from build123d import *

# Parameters (mm, degrees)
EXTRUDE_1_DEPTH        = 5
SKETCH_1_4_OUTSIDE_W   = 152.016
SKETCH_1_4_OUTSIDE_H   = 122.016
SKETCH_1_4_OUTSIDE_R   = 1.7
SKETCH_1_4_OUTSIDE_R_2 = 1.6
CUT_EXTRUDE_3_DEPTH    = 84.683501662
SKETCH_2_W             = 7.5
SKETCH_2_H             = 25
EXTRUDE_2_DEPTH        = 20
FILLET_1_R             = 2
SKETCH_6_R             = 1.6
CUT_EXTRUDE_4_DEPTH    = 7.5
SKETCH_7_R             = 1.6
CUT_EXTRUDE_5_DEPTH    = 134.554368416


with BuildPart() as part:
    # 스케치1 → 보스-돌출1 (new body)
    with BuildSketch(Plane.XY):
        with BuildLine():
            Line((-57.749377558, 34.859778143), (52.250622442, 34.859778143))
            ThreePointArc((52.250622442, 34.859778143), (55.786156348, 33.395312049), (57.250622442, 29.859778143))
            Line((57.250622442, 29.859778143), (57.250622442, -50.140221857))
            ThreePointArc((57.250622442, -50.140221857), (55.786156348, -53.675755763), (52.250622442, -55.140221857))
            Line((52.250622442, -55.140221857), (-57.749377558, -55.140221857))
            ThreePointArc((-57.749377558, -55.140221857), (-61.284911464, -53.675755763), (-62.749377558, -50.140221857))
            Line((-62.749377558, -50.140221857), (-62.749377558, 29.859778143))
            ThreePointArc((-62.749377558, 29.859778143), (-61.284911464, 33.395312049), (-57.749377558, 34.859778143))
        make_face()
    extrude(amount=-EXTRUDE_1_DEPTH)

    # 스케치1<4> outside → 컷-돌출3 (cut, through all)
    # profile 1 of 11: a face of its own
    with BuildSketch(Plane.XY):
        with Locations((-2.749, -10.14)):
            Rectangle(SKETCH_1_4_OUTSIDE_W, SKETCH_1_4_OUTSIDE_H)
        with BuildLine():
            Line((-57.749377558, 34.859778143), (52.250622442, 34.859778143))
            ThreePointArc((52.250622442, 34.859778143), (55.786156348, 33.395312049), (57.250622442, 29.859778143))
            Line((57.250622442, 29.859778143), (57.250622442, -50.140221857))
            ThreePointArc((57.250622442, -50.140221857), (55.786156348, -53.675755763), (52.250622442, -55.140221857))
            Line((52.250622442, -55.140221857), (-57.749377558, -55.140221857))
            ThreePointArc((-57.749377558, -55.140221857), (-61.284911464, -53.675755763), (-62.749377558, -50.140221857))
            Line((-62.749377558, -50.140221857), (-62.749377558, 29.859778143))
            ThreePointArc((-62.749377558, 29.859778143), (-61.284911464, 33.395312049), (-57.749377558, 34.859778143))
        make_face(mode=Mode.SUBTRACT)
    # profile 2 of 11: a face of its own
    with BuildSketch(Plane.XY):
        with Locations((-57.749377558, 29.859778143)):
            Circle(SKETCH_1_4_OUTSIDE_R)
    # profile 3 of 11: a face of its own
    with BuildSketch(Plane.XY):
        with Locations((52.250622442, 29.859778143)):
            Circle(SKETCH_1_4_OUTSIDE_R)
    # profile 4 of 11: a face of its own
    with BuildSketch(Plane.XY):
        with Locations((-57.749377558, -50.140221857)):
            Circle(SKETCH_1_4_OUTSIDE_R)
    # profile 5 of 11: a face of its own
    with BuildSketch(Plane.XY):
        with Locations((52.250622442, -50.140221857)):
            Circle(SKETCH_1_4_OUTSIDE_R)
    # profile 6 of 11: a face of its own
    with BuildSketch(Plane.XY):
        with Locations((-47.749377558, 9.859778143)):
            Circle(SKETCH_1_4_OUTSIDE_R)
    # profile 7 of 11: a face of its own
    with BuildSketch(Plane.XY):
        with Locations((-47.749377558, -30.140221857)):
            Circle(SKETCH_1_4_OUTSIDE_R)
    # profile 8 of 11: a face of its own
    with BuildSketch(Plane.XY):
        with Locations((42.250622442, 9.859778143)):
            Circle(SKETCH_1_4_OUTSIDE_R)
    # profile 9 of 11: a face of its own
    with BuildSketch(Plane.XY):
        with Locations((42.250622442, -30.140221857)):
            Circle(SKETCH_1_4_OUTSIDE_R)
    # profile 10 of 11: a face of its own
    with BuildSketch(Plane.XY):
        with Locations((-2.74831555, -0.140221857)):
            Circle(SKETCH_1_4_OUTSIDE_R_2)
    # profile 11 of 11: a face of its own
    with BuildSketch(Plane.XY):
        with Locations((-2.74831555, -20.140221857)):
            Circle(SKETCH_1_4_OUTSIDE_R_2)
    extrude(amount=-CUT_EXTRUDE_3_DEPTH, mode=Mode.SUBTRACT)

    # 스케치2 → 보스-돌출2 (add)
    with BuildSketch(Plane.XY):
        with Locations((-58.999377558, -10.043662602)):
            Rectangle(SKETCH_2_W, SKETCH_2_H)
        with Locations((53.485310034, -10.043662602)):
            Rectangle(SKETCH_2_W, SKETCH_2_H)
    extrude(amount=EXTRUDE_2_DEPTH)

    # 필렛1
    fillet_1_edges = [part.edges().sort_by_distance(p)[0] for p in [
        (-58.999377558, -22.543662602, 20),
        (-58.999377558, 2.456337398, 20),
        (53.485310034, 2.456337398, 20),
        (53.485310034, -22.543662602, 20),
    ]]
    fillet(fillet_1_edges, radius=FILLET_1_R)

    # 스케치6 → 컷-돌출4 (cut)
    with BuildSketch(Plane.ZY.offset(62.749377558)):
        with Locations(Location((5, -18.843662602, 0), (0, 0, 270))):
            Circle(SKETCH_6_R)
        with Locations(Location((5, -1.243662602, 0), (0, 0, 270))):
            Circle(SKETCH_6_R)
    extrude(amount=-CUT_EXTRUDE_4_DEPTH, mode=Mode.SUBTRACT)

    # 스케치7 → 컷-돌출5 (cut, through all)
    with BuildSketch(Plane(origin=(57.235310034, 0, 0), x_dir=(0, 0, -1), z_dir=(1, 0, 0))):
        with Locations(Location((-5, -1.243662602, 0), (0, 0, 270))):
            Circle(SKETCH_7_R)
        with Locations(Location((-5, -18.843662602, 0), (0, 0, 270))):
            Circle(SKETCH_7_R)
    extrude(amount=-CUT_EXTRUDE_5_DEPTH, mode=Mode.SUBTRACT)


solid = part.part
Verification items for the finished model (mm, model axes). A direction names the side the tool comes from. Give positions to 0.01 mm unless a question says otherwise; leave off trailing zeros. Loops run counter-clockwise (first coordinate to the right, second up) from the corner with the lowest first, then second, coordinate; pieces in that order, holes last.
1) Sectioned sample at B-B, the plane z = 5. Enter the section's corners in (x, y), then the cut area to 3 significant figures.
2) Sectioned sample at A-A, the plane z = 12.75. Enter the section's corners in (x, y).
3) Depth check by flat-ended pin: pin 1 Ø10 at (y, z) = (-11, 6.5) entering from +X; pin 2 Ø3 at (x, y) = (-2.75, -20.14) entering from +Z; pin 3 Ø6 at (x, z) = (53, 9.5) entering from -Y; pin 4 Ø6 at (x, y) = (32, -34) entering from +Z. Enter the tip coordinate at first touch or a pass-through.
4) Thickness scan on line 1 along X through (y, z) = (-16.5, 15); line 2 along Z through (x, y) = (23, 18). Record the ranges inside material, lowest first.
5) Sectioned sample at D-D, the plane y = 18. Enter the section's corners in (x, z).
6) Draft check along Y on faces 1 (the cylindrical face through (55.82, -53.64, -2.46)), 2 (the cylindrical face through (-49.448, 9.935, -2.465)), 3 (the flat face through (53, 2.456, 9)). Enter one of: pulls with the +Y half, pulls with the -Y half, needs draft (parallel to the pull), parting line crosses it, or undercut.
7) Sectioned sample at C-C, the plane x = -7.5. Enter the section's corners in (y, z).
8) Set-up check for faces 4 (the cylindrical face through (-59, -48.99, -2.46)), 5 (the flat face through (53, -22.544, 9)), 6 (the flat face through (-55.249, -10, 10)): record each of +Z, -Z, +X, -X, +Y, -Y from which the full face is reachable in a straight line by a thin tool's end or side.
Answers:
1. outline: (-62.75, -22.54) - (-55.25, -22.54) - (-55.25, -20.44) - (-62.75, -20.44) - close; (-62.75, -17.24) - (-55.25, -17.24) - (-55.25, -2.84) - (-62.75, -2.84) - close; (-62.75, 0.36) - (-55.25, 0.36) - (-55.25, 2.46) - (-62.75, 2.46) - close; (49.74, -22.54) - (57.24, -22.54) - (57.24, -20.44) - (49.74, -20.44) - close; (49.74, -17.24) - (57.24, -17.24) - (57.24, -2.84) - (49.74, -2.84) - close; (49.74, 0.36) - (57.24, 0.36) - (57.24, 2.46) - (49.74, 2.46) - close
1. area: 279 mm2
2. outline: (-62.75, -22.54) - (-55.25, -22.54) - (-55.25, 2.46) - (-62.75, 2.46) - close; (49.74, -22.54) - (57.24, -22.54) - (57.24, 2.46) - (49.74, 2.46) - close
3. pin 1: stops at x = 57.24
3. pin 2: passes through
3. pin 3: stops at y = -22.54
3. pin 4: stops at z = 0
4. line 1: x = -62.75 to -55.25, 49.74 to 57.24
4. line 2: z = -5 to 0
5. outline: (-62.75, -5) - (57.25, -5) - (57.25, 0) - (-62.75, 0) - close
6. face 1: pulls with the -Y half
6. face 2: undercut
6. face 3: pulls with the +Y half
7. outline: (-55.14, -5) - (34.86, -5) - (34.86, 0) - (-55.14, 0) - close
8. face 4: +Z, -Z
8. face 5: +Z, +X, -X, -Y
8. face 6: +Z, +Y, -Y
